The listing builds one solid part. Answer for the finished solid, in the listing's coordinates (mm). Coordinates: 2 decimals unless noted, no trailing zeros. Write each loop counter-clockwise with the first axis right and the second up, starting at its lowest first coordinate (ties: lowest second). Pieces come first, ordered by that corner, then holes.
from build123d import *

# Parameters (mm, degrees)
SKETCH1_W                                           = 12.7
SKETCH1_H                                           = 279.4
BOSS_EXTRUDE1_DEPTH                                 = 93.98
SKETCH2_R                                           = 2.0828
SKETCH2_R_2                                         = 1.778
CUT_EXTRUDE1_DEPTH                                  = 13.7
CBORE_FOR_8_BINDING_HEAD_MACHINE_SCREW1_D           = 4.4958
CBORE_FOR_8_BINDING_HEAD_MACHINE_SCREW1_CBORE_D     = 9.525
CBORE_FOR_8_BINDING_HEAD_MACHINE_SCREW1_CBORE_DEPTH = 2.667
F_1_4_20_TAPPED_HOLE1_D                             = 5.1054
F_1_4_20_TAPPED_HOLE1_DEPTH                         = 25.4
F_1_4_20_TAPPED_HOLE1_TIP                           = 1.533816902


with BuildPart() as part:
    # Sketch1 → Boss-Extrude1 (new body)
    with BuildSketch(Plane(origin=(0, 0, 0), x_dir=(1, 0, 0), z_dir=(0, 1, 0))):
        with Locations((6.35, -139.7)):
            Rectangle(SKETCH1_W, SKETCH1_H)
    extrude(amount=BOSS_EXTRUDE1_DEPTH)

    # Sketch2 → Cut-Extrude1 (cut, through all)
    with BuildSketch(Plane(origin=(12.7, 0, 0), x_dir=(0, 0, -1), z_dir=(1, 0, 0))):
        with Locations((-246.38, 84.836)):
            Circle(SKETCH2_R)
        with Locations((-231.14, 84.836)):
            Circle(SKETCH2_R)
        with BuildLine():
            ThreePointArc((-236.982, 77.216), (-238.76, 78.994), (-240.538, 77.216))
            Line((-240.538, 77.216), (-236.982, 77.216))
        make_face()
        with BuildLine():
            Line((-236.982, 77.216), (-240.538, 77.216))
            ThreePointArc((-240.538, 77.216), (-238.76, 75.438), (-236.982, 77.216))
        make_face()
        with Locations((-246.38, 69.596)):
            Circle(SKETCH2_R)
        with Locations((-231.14, 69.596)):
            Circle(SKETCH2_R)
        with BuildLine():
            ThreePointArc((-176.022, 77.216), (-177.8, 78.994), (-179.578, 77.216))
            Line((-179.578, 77.216), (-176.022, 77.216))
        make_face()
        with BuildLine():
            Line((-176.022, 77.216), (-179.578, 77.216))
            ThreePointArc((-179.578, 77.216), (-177.8, 75.438), (-176.022, 77.216))
        make_face()
        with Locations((-185.42, 84.836)):
            Circle(SKETCH2_R)
        with Locations((-170.18, 84.836)):
            Circle(SKETCH2_R)
        with Locations((-170.18, 69.596)):
            Circle(SKETCH2_R)
        with Locations((-185.42, 69.596)):
            Circle(SKETCH2_R)
        with BuildLine():
            ThreePointArc((-99.822, 77.216), (-101.6, 78.994), (-103.378, 77.216))
            Line((-103.378, 77.216), (-99.822, 77.216))
        make_face()
        with BuildLine():
            Line((-99.822, 77.216), (-103.378, 77.216))
            ThreePointArc((-103.378, 77.216), (-101.6, 75.438), (-99.822, 77.216))
        make_face()
        with Locations((-109.22, 69.596)):
            Circle(SKETCH2_R)
        with Locations((-93.98, 84.836)):
            Circle(SKETCH2_R)
        with Locations((-109.22, 84.836)):
            Circle(SKETCH2_R)
        with Locations((-48.26, 69.596)):
            Circle(SKETCH2_R)
        with Locations((-48.26, 84.836)):
            Circle(SKETCH2_R)
        with Locations((-33.02, 84.836)):
            Circle(SKETCH2_R)
        with Locations((-33.02, 69.596)):
            Circle(SKETCH2_R)
        with Locations((-93.98, 69.596)):
            Circle(SKETCH2_R)
        with Locations((-40.64, 77.216)):
            Circle(SKETCH2_R_2)
    extrude(amount=-CUT_EXTRUDE1_DEPTH, mode=Mode.SUBTRACT)

    # CBORE for #8 Binding Head Machine Screw1 (through all)
    with Locations(Plane.ZY):
        with Locations((246.38, 84.836), (246.38, 69.596), (231.14, 69.596), (231.14, 84.836), (185.42, 69.596), (185.42, 84.836), (170.18, 84.836), (170.18, 69.596), (109.22, 69.596), (93.98, 69.596), (93.98, 84.836), (109.22, 84.836), (48.26, 69.596), (33.02, 69.596), (33.02, 84.836), (48.26, 84.836)):
            CounterBoreHole(CBORE_FOR_8_BINDING_HEAD_MACHINE_SCREW1_D / 2, CBORE_FOR_8_BINDING_HEAD_MACHINE_SCREW1_CBORE_D / 2, CBORE_FOR_8_BINDING_HEAD_MACHINE_SCREW1_CBORE_DEPTH)

    # 1/4-20 Tapped Hole1
    with Locations(Plane(origin=(0, 0, 0), x_dir=(-1, 0, 0), z_dir=(0, -1, 0))):
        with Locations((-6.35, -25.4), (-6.35, -101.6), (-6.35, -177.8), (-6.35, -254)):
            Hole(F_1_4_20_TAPPED_HOLE1_D / 2, depth=F_1_4_20_TAPPED_HOLE1_DEPTH)
            with Locations((0, 0, -(F_1_4_20_TAPPED_HOLE1_DEPTH + F_1_4_20_TAPPED_HOLE1_TIP / 2))):  # 118° drill point
                Cone(0, F_1_4_20_TAPPED_HOLE1_D / 2, F_1_4_20_TAPPED_HOLE1_TIP, mode=Mode.SUBTRACT)


solid = part.part
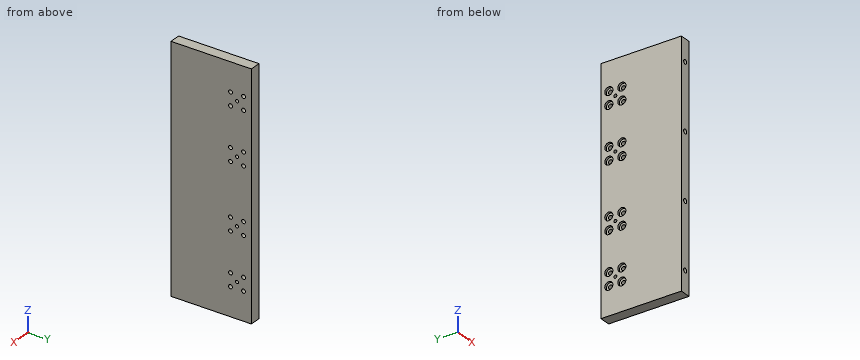
Q1. Given pin 1 (3 mm diameter, centred on y = 67.5, z = 245.5, fed in from -X), flat-ended and moving along its own axis, determine where the tip first touches the part or whether it passes through.
Answers below:
pin 1: stops at x = 2.67
Q2. Find the intervals of material crossed by probe 1 along Y at (x, z) = (8.25, 93.98); probe 2 along X at (y, z) = (67, 171); probe 3 along Y at (x, z) = (6, 252.5), in increasing order.
Answers below:
probe 1: y = 0 to 67.35, 71.84 to 82.59, 87.08 to 93.98
probe 2: x = 2.67 to 12.7
probe 3: y = 26.01 to 93.98
Q3. The part is cut by section A-A, the plane y = 10. Write down the section's boundary in (x, z), then the cut area to 3 significant figures.
Answers below:
outline: (0, 0) - (12.7, 0) - (12.7, 279.4) - (0, 279.4) - close; hole circle Ø5.11 at (6.35, 25.4); hole circle Ø5.11 at (6.35, 101.6); hole circle Ø5.11 at (6.35, 177.8); hole circle Ø5.11 at (6.35, 254)
area: 3,470 mm2
